Source: CAD feature listing. Evaluate the final solid. Frame: model axes, mm. Give positions to 0.01 mm unless a question says otherwise; leave off trailing zeros. Order: outer loops, then holes, each group sorted by start corner. A loop starts at its lowest first (then second) coordinate and runs counter-clockwise, first axis right, second up. Notation, with made-up numbers: (37.5, 46) - (62.5, 46) arc R27 cw to (62.5, 64) - close; hole circle Ø5 at (67.25, 65). An arc over 180 degrees is marked (long way). Write each question's results on one line, items separated by ' | '. Start each with the question number.
Item 1: Mould query, pull axis Z, two halves, no side actions, for faces 1 (the flat face through (97, 3.17, -102)), 2 (the flat face through (10, 2, -39)), 3 (the flat face through (96.628, 1.607, -5.998)), 4 (the flat face through (186, 2, -39)). Classes: released by +Z, released by -Z, zero draft, split by the parting line, or undercut.
Item 2: Section A-A on y = 1.05. State how many separate pieces and enclosed holes the cut face has, and give its area (3 significant figures).
Item 3: Section C-C on x = 127.5. Output: boundary loops of the cut face in (y, z).
Item 4: Contact query for flat-ended pins moving along their axis: pin 1 Ø1.3 at (y, z) = (2.5, -36.5) entering from -X; pin 2 Ø2.5 at (x, z) = (111.5, -185) entering from +Y; pin 3 Ø3.5 at (x, z) = (185.5, -42.01) entering from +Y; pin 4 Ø1.6 at (x, y) = (17, 1) entering from -Z. Output: stop coordinate, or through.
Item 5: Line query: line 1 along X through (y, z) = (1.45, -42.01); line 2 along X through (y, z) = (1.4, -185) (3 decimals); line 3 along X through (y, z) = (1.65, -138.5). Output: solid intervals per line, ascending.
Item 6: Section B-B on x = 29. Output: boundary loops of the cut face in (y, z).
```python
from build123d import *

# Parameters (mm, degrees)
SALIENTE_EXTRUIR1_DEPTH = 196
CORTAR_EXTRUIR1_REACH   = 274.995
CROQUIS2_W              = 37.5
CROQUIS2_H              = 62.989872981
CROQUIS3_W              = 13
CROQUIS3_H              = 22.5
CORTAR_EXTRUIR2_DEPTH   = 1.17
CORTAR_EXTRUIR3_REACH   = 274.984
CROQUIS5_W              = 7.25
CROQUIS5_H              = 7.25
CORTAR_EXTRUIR4_REACH   = 274.984
CROQUIS6_R              = 1.6
CUT_EXTRUDE1_REACH      = 274.995
SKETCH1_R               = 1.585
CUT_EXTRUDE2_REACH      = 274.995
SKETCH2_R               = 1.585
CUT_EXTRUDE3_REACH      = 274.995
SKETCH3_R               = 1.579889923
SKETCH3_R_2             = 1.585


with BuildPart() as part:
    # Croquis1 → Saliente-Extruir1 (new body)
    with BuildSketch(Plane(origin=(0, 0, 0), x_dir=(0, 0, -1), z_dir=(1, 0, 0))):
        Polygon((0, 0), (190, 0), (190, 3.17), (11.83060106, 3.17), align=None)
    extrude(amount=SALIENTE_EXTRUIR1_DEPTH)

    # Croquis2 → Cortar-Extruir1 (cut, up to next)
    with BuildSketch(Plane(origin=(0, 0, 0), x_dir=(-1, 0, 0), z_dir=(0, -1, 0)), mode=Mode.PRIVATE) as cortar_extruir1_sk1:
        with Locations((-18.75, 158.50506351)):
            Rectangle(CROQUIS2_W, CROQUIS2_H)
    cortar_extruir1_tool1 = extrude(cortar_extruir1_sk1.sketch, amount=-CORTAR_EXTRUIR1_REACH, mode=Mode.PRIVATE) & part.part
    cortar_extruir1 = cortar_extruir1_tool1.solids().sort_by_distance((18.75, 0, -158.505064))[0]
    add(cortar_extruir1, mode=Mode.SUBTRACT)

    # Simetría1: Cortar-Extruir1 across plane
    add(cortar_extruir1.mirror(Plane.ZY.offset(-98)), mode=Mode.SUBTRACT)

    # Croquis3 → Cortar-Extruir2 (cut)
    with BuildSketch(Plane(origin=(0, 3.17, 0), x_dir=(1, 0, 0), z_dir=(0, 1, 0))):
        with Locations((10.5, 36.41)):
            Rectangle(CROQUIS3_W, CROQUIS3_H)
    cortar_extruir2 = extrude(amount=-CORTAR_EXTRUIR2_DEPTH, mode=Mode.SUBTRACT)

    # Croquis5 → Cortar-Extruir3 (cut, up to next)
    with BuildSketch(Plane(origin=(0, 2, 0), x_dir=(1, 0, 0), z_dir=(0, 1, 0)), mode=Mode.PRIVATE) as cortar_extruir3_sk1:
        with Locations((10.5, 30.035)):
            Rectangle(CROQUIS5_W, CROQUIS5_H)
    cortar_extruir3_tool1 = extrude(cortar_extruir3_sk1.sketch, amount=-CORTAR_EXTRUIR3_REACH, mode=Mode.PRIVATE) & part.part
    cortar_extruir3 = cortar_extruir3_tool1.solids().sort_by_distance((10.5, 2, -30.035))[0]
    add(cortar_extruir3, mode=Mode.SUBTRACT)

    # Croquis6 → Cortar-Extruir4 (cut, up to next)
    with BuildSketch(Plane(origin=(0, 2, 0), x_dir=(1, 0, 0), z_dir=(0, 1, 0)), mode=Mode.PRIVATE) as cortar_extruir4_sk1:
        with Locations(Location((10.5, 42.01, 0), (0, 0, 270))):
            Circle(CROQUIS6_R)
    cortar_extruir4_tool1 = extrude(cortar_extruir4_sk1.sketch, amount=-CORTAR_EXTRUIR4_REACH, mode=Mode.PRIVATE) & part.part
    cortar_extruir4 = cortar_extruir4_tool1.solids().sort_by_distance((10.5, 2, -42.01))[0]
    add(cortar_extruir4, mode=Mode.SUBTRACT)

    # Simetría2: Cortar-Extruir2, Cortar-Extruir3, Cortar-Extruir4 across plane
    add(cortar_extruir2.mirror(Plane.ZY.offset(-98)), mode=Mode.SUBTRACT)
    add(cortar_extruir3.mirror(Plane.ZY.offset(-98)), mode=Mode.SUBTRACT)
    add(cortar_extruir4.mirror(Plane.ZY.offset(-98)), mode=Mode.SUBTRACT)

    # Sketch1 → Cut-Extrude1 (cut, up to next)
    with BuildSketch(Plane(origin=(0, 3.17, 0), x_dir=(1, 0, 0), z_dir=(0, 1, 0)), mode=Mode.PRIVATE) as cut_extrude1_sk1:
        with Locations(Location((8.5, 118.010127019, 0), (0, 0, 270))):
            Circle(SKETCH1_R)
    cut_extrude1_tool1 = extrude(cut_extrude1_sk1.sketch, amount=-CUT_EXTRUDE1_REACH, mode=Mode.PRIVATE) & part.part
    # Sketch1 → Cut-Extrude1 (cut, up to next)
    with BuildSketch(Plane(origin=(0, 3.17, 0), x_dir=(1, 0, 0), z_dir=(0, 1, 0)), mode=Mode.PRIVATE) as cut_extrude1_sk2:
        with Locations(Location((187.5, 118.010127019, 0), (0, 0, 270))):
            Circle(SKETCH1_R)
    cut_extrude1_tool2 = extrude(cut_extrude1_sk2.sketch, amount=-CUT_EXTRUDE1_REACH, mode=Mode.PRIVATE) & part.part
    add(cut_extrude1_tool1.solids().sort_by_distance((8.5, 3.17, -118.010127))[0], mode=Mode.SUBTRACT)
    add(cut_extrude1_tool2.solids().sort_by_distance((187.5, 3.17, -118.010127))[0], mode=Mode.SUBTRACT)

    # Sketch2 → Cut-Extrude2 (cut, up to next)
    with BuildSketch(Plane(origin=(0, 3.17, 0), x_dir=(1, 0, 0), z_dir=(0, 1, 0)), mode=Mode.PRIVATE) as cut_extrude2_sk1:
        with Locations(Location((98.5, 38.010127019, 0), (0, 0, 270))):
            Circle(SKETCH2_R)
    cut_extrude2_tool1 = extrude(cut_extrude2_sk1.sketch, amount=-CUT_EXTRUDE2_REACH, mode=Mode.PRIVATE) & part.part
    add(cut_extrude2_tool1.solids().sort_by_distance((98.5, 3.17, -38.010127))[0], mode=Mode.SUBTRACT)

    # Sketch3 → Cut-Extrude3 (cut, up to next)
    with BuildSketch(Plane(origin=(0, 3.17, 0), x_dir=(1, 0, 0), z_dir=(0, 1, 0)), mode=Mode.PRIVATE) as cut_extrude3_sk1:
        with Locations(Location((43.5, 185, 0), (0, 0, 270))):
            Circle(SKETCH3_R)
    cut_extrude3_tool1 = extrude(cut_extrude3_sk1.sketch, amount=-CUT_EXTRUDE3_REACH, mode=Mode.PRIVATE) & part.part
    # Sketch3 → Cut-Extrude3 (cut, up to next)
    with BuildSketch(Plane(origin=(0, 3.17, 0), x_dir=(1, 0, 0), z_dir=(0, 1, 0)), mode=Mode.PRIVATE) as cut_extrude3_sk2:
        with Locations(Location((84.5, 185, 0), (0, 0, 270))):
            Circle(SKETCH3_R_2)
    cut_extrude3_tool2 = extrude(cut_extrude3_sk2.sketch, amount=-CUT_EXTRUDE3_REACH, mode=Mode.PRIVATE) & part.part
    # Sketch3 → Cut-Extrude3 (cut, up to next)
    with BuildSketch(Plane(origin=(0, 3.17, 0), x_dir=(1, 0, 0), z_dir=(0, 1, 0)), mode=Mode.PRIVATE) as cut_extrude3_sk3:
        with Locations(Location((152.5, 185, 0), (0, 0, 270))):
            Circle(SKETCH3_R_2)
    cut_extrude3_tool3 = extrude(cut_extrude3_sk3.sketch, amount=-CUT_EXTRUDE3_REACH, mode=Mode.PRIVATE) & part.part
    # Sketch3 → Cut-Extrude3 (cut, up to next)
    with BuildSketch(Plane(origin=(0, 3.17, 0), x_dir=(1, 0, 0), z_dir=(0, 1, 0)), mode=Mode.PRIVATE) as cut_extrude3_sk4:
        with Locations(Location((111.5, 185, 0), (0, 0, 270))):
            Circle(SKETCH3_R_2)
    cut_extrude3_tool4 = extrude(cut_extrude3_sk4.sketch, amount=-CUT_EXTRUDE3_REACH, mode=Mode.PRIVATE) & part.part
    # Sketch3 → Cut-Extrude3 (cut, up to next)
    with BuildSketch(Plane(origin=(0, 3.17, 0), x_dir=(1, 0, 0), z_dir=(0, 1, 0)), mode=Mode.PRIVATE) as cut_extrude3_sk5:
        with Locations(Location((111.5, 136.5, 0), (0, 0, 270))):
            Circle(SKETCH3_R_2)
    cut_extrude3_tool5 = extrude(cut_extrude3_sk5.sketch, amount=-CUT_EXTRUDE3_REACH, mode=Mode.PRIVATE) & part.part
    # Sketch3 → Cut-Extrude3 (cut, up to next)
    with BuildSketch(Plane(origin=(0, 3.17, 0), x_dir=(1, 0, 0), z_dir=(0, 1, 0)), mode=Mode.PRIVATE) as cut_extrude3_sk6:
        with Locations(Location((152.5, 136.5, 0), (0, 0, 270))):
            Circle(SKETCH3_R_2)
    cut_extrude3_tool6 = extrude(cut_extrude3_sk6.sketch, amount=-CUT_EXTRUDE3_REACH, mode=Mode.PRIVATE) & part.part
    # Sketch3 → Cut-Extrude3 (cut, up to next)
    with BuildSketch(Plane(origin=(0, 3.17, 0), x_dir=(1, 0, 0), z_dir=(0, 1, 0)), mode=Mode.PRIVATE) as cut_extrude3_sk7:
        with Locations(Location((84.5, 136.5, 0), (0, 0, 270))):
            Circle(SKETCH3_R_2)
    cut_extrude3_tool7 = extrude(cut_extrude3_sk7.sketch, amount=-CUT_EXTRUDE3_REACH, mode=Mode.PRIVATE) & part.part
    # Sketch3 → Cut-Extrude3 (cut, up to next)
    with BuildSketch(Plane(origin=(0, 3.17, 0), x_dir=(1, 0, 0), z_dir=(0, 1, 0)), mode=Mode.PRIVATE) as cut_extrude3_sk8:
        with Locations(Location((43.5, 136.5, 0), (0, 0, 270))):
            Circle(SKETCH3_R_2)
    cut_extrude3_tool8 = extrude(cut_extrude3_sk8.sketch, amount=-CUT_EXTRUDE3_REACH, mode=Mode.PRIVATE) & part.part
    add(cut_extrude3_tool1.solids().sort_by_distance((43.5, 3.17, -185))[0], mode=Mode.SUBTRACT)
    add(cut_extrude3_tool2.solids().sort_by_distance((84.5, 3.17, -185))[0], mode=Mode.SUBTRACT)
    add(cut_extrude3_tool3.solids().sort_by_distance((152.5, 3.17, -185))[0], mode=Mode.SUBTRACT)
    add(cut_extrude3_tool4.solids().sort_by_distance((111.5, 3.17, -185))[0], mode=Mode.SUBTRACT)
    add(cut_extrude3_tool5.solids().sort_by_distance((111.5, 3.17, -136.5))[0], mode=Mode.SUBTRACT)
    add(cut_extrude3_tool6.solids().sort_by_distance((152.5, 3.17, -136.5))[0], mode=Mode.SUBTRACT)
    add(cut_extrude3_tool7.solids().sort_by_distance((84.5, 3.17, -136.5))[0], mode=Mode.SUBTRACT)
    add(cut_extrude3_tool8.solids().sort_by_distance((43.5, 3.17, -136.5))[0], mode=Mode.SUBTRACT)


solid = part.part
```
Evaluation:
1) face 1: zero draft | face 2: undercut | face 3: released by +Z | face 4: undercut
2) separate pieces: 1 | enclosed holes: 15 | area: 31,500 mm^2
3) outline: (0, -190) - (3.17, -190) - (3.17, -11.83) - (0, 0) - close
4) pin 1: stops at x = 0 | pin 2: passes through | pin 3: stops at y = 2 | pin 4: stops at z = -127.01
5) line 1: x = 0 to 8.9, 12.1 to 183.9, 187.1 to 196 | line 2: x = 37.5 to 41.92, 45.08 to 82.915, 86.085 to 109.915, 113.085 to 150.915, 154.085 to 158.5 | line 3: x = 37.5 to 158.5
6) outline: (0, -127.01) - (3.17, -127.01) - (3.17, -11.83) - (0, 0) - close
